Print and shaded views of the part. All mm, measured from the part's lowest x, y and z. Give positions to 0.01 mm unless a question says otherwise; leave off trailing zeros. Write each loop counter-clockwise with the first axis right and the second up, starting at its lowest first coordinate (ties: lowest second). Pieces come first, ordered by that corner, then holes.
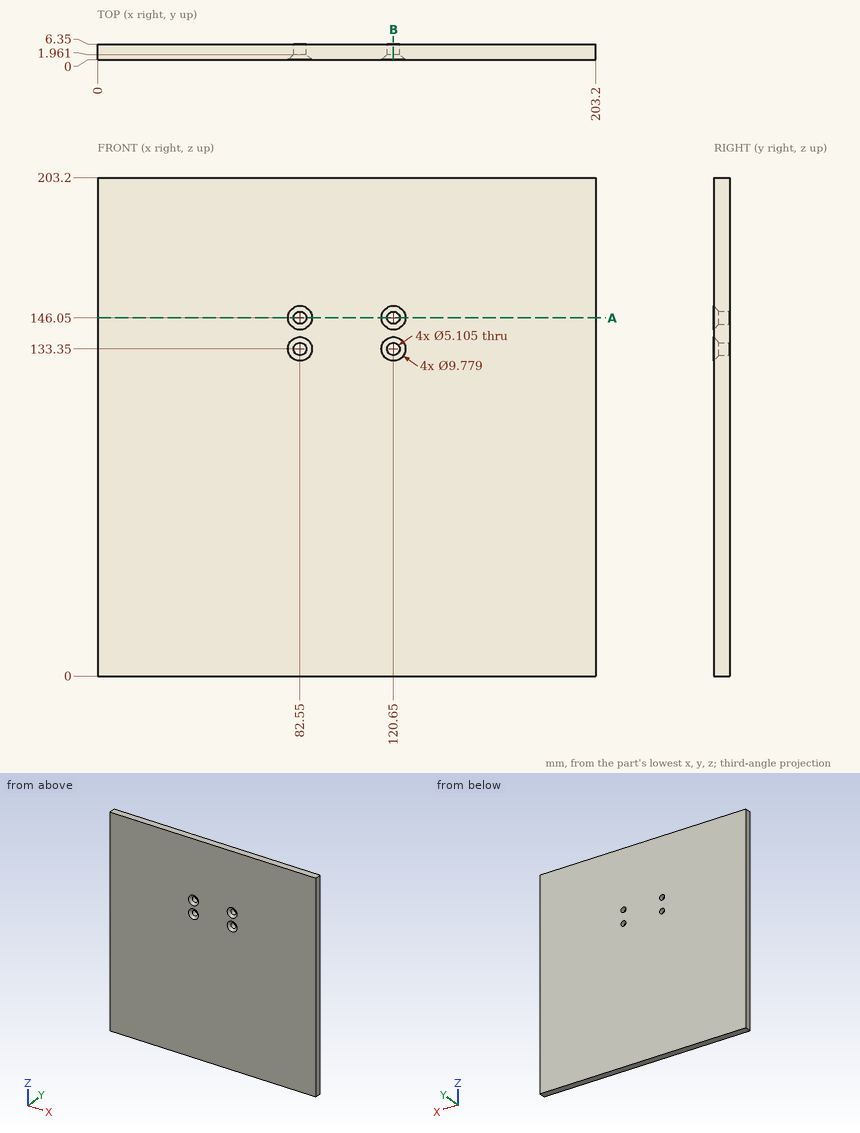
1. Drill centre lines: line 1 along X through (y, z) = (5.2, 133.35); line 2 along Z through (x, y) = (82.55, 4.85); line 3 along X through (y, z) = (5, 135). Where is each one in solid material? Low to high.
2. Saw through at A-A on z = 146.05. Give the cut face in (x, y), plus the area to 3 significant figures.
3. Saw through at B-B on x = 120.65. Give the cut face in (y, z).
4. Drop flat-ended pins along their axis: pin 1 (2 mm diameter, centred on y = 2.5, z = 121.5, fed in from -X); pin 2 (8 mm diameter, centred on x = 82.55, z = 133.35, fed in from -Y) (1 decimal). Give the stop position or say it passes through.
Outcome:
1. line 1: x = 0 to 80, 85.1 to 118.1, 123.2 to 203.2
1. line 2: z = 0 to 130.8, 135.9 to 143.5, 148.6 to 203.2
1. line 3: x = 0 to 80.6, 84.5 to 118.7, 122.6 to 203.2
2. outline: (0, 0) - (77.66, 0) - (80, 1.96) - (80, 6.35) - (0, 6.35) - close; (85.1, 1.96) - (87.44, 0) - (115.76, 0) - (118.1, 1.96) - (118.1, 6.35) - (85.1, 6.35) - close; (123.2, 1.96) - (125.54, 0) - (203.2, 0) - (203.2, 6.35) - (123.2, 6.35) - close
2. area: 1,220 mm2
3. outline: (0, 0) - (6.35, 0) - (6.35, 130.8) - (1.96, 130.8) - (0, 128.46) - close; (0, 138.24) - (1.96, 135.9) - (6.35, 135.9) - (6.35, 143.5) - (1.96, 143.5) - (0, 141.16) - close; (0, 150.94) - (1.96, 148.6) - (6.35, 148.6) - (6.35, 203.2) - (0, 203.2) - close
4. pin 1: stops at x = 0
4. pin 2: stops at y = 0.7
